```python
from build123d import *

# Parameters (mm, degrees)
BOSS_EXTRUDE1_DEPTH      = 150
BOSS_EXTRUDE1_DEPTH_BACK = 150
SKETCH2_W                = 600
SKETCH2_H                = 200
SKETCH3_W                = 200
SKETCH3_H                = 100
CUT_EXTRUDE1_DEPTH       = 100
SKETCH4_W                = 25
SKETCH4_H                = 25
BOSS_EXTRUDE2_DEPTH      = 5
MIRROR3_COPY_1_SKETCH_W  = 25
MIRROR3_COPY_1_SKETCH_H  = 25
MIRROR3_COPY_1_DEPTH     = 5
CUT_EXTRUDE3_DEPTH       = 200


with BuildPart() as part:
    # Sketch2 → Boss-Extrude1 (new, two sides: drawn at the far end of the back side and taken through both)
    with BuildSketch(Plane(origin=(0, 0, 0), x_dir=(0, 0, -1), z_dir=(1, 0, 0)).offset(-BOSS_EXTRUDE1_DEPTH_BACK)):
        Rectangle(SKETCH2_W, SKETCH2_H)
    extrude(amount=BOSS_EXTRUDE1_DEPTH + BOSS_EXTRUDE1_DEPTH_BACK)

    # Sketch3 → Cut-Extrude1 (cut)
    with BuildSketch(Plane(origin=(150, 0, 0), x_dir=(0, 0, -1), z_dir=(1, 0, 0))):
        with Locations((-200, -50)):
            Rectangle(SKETCH3_W, SKETCH3_H)
        with Locations((200, -50)):
            Rectangle(SKETCH3_W, SKETCH3_H)
    cut_extrude1 = extrude(amount=-CUT_EXTRUDE1_DEPTH, mode=Mode.SUBTRACT)

    # Mirror1: Cut-Extrude1 across plane
    add(cut_extrude1.mirror(Plane(origin=(0, 0, 0), x_dir=(0, 0, 1), z_dir=(1, 0, 0))), mode=Mode.SUBTRACT)

    # Sketch4 → Boss-Extrude2 (add)
    with BuildSketch(Plane.XZ):
        with Locations((112.5, 212.5)):
            Rectangle(SKETCH4_W, SKETCH4_H)
    boss_extrude2 = extrude(amount=BOSS_EXTRUDE2_DEPTH)

    # Mirror2: Boss-Extrude2 across plane
    add(boss_extrude2.mirror(Plane(origin=(0, 0, 0), x_dir=(0, 0, 1), z_dir=(1, 0, 0))))

    # Mirror3: Boss-Extrude2 across plane
    add(boss_extrude2.mirror(Plane.XY))

    # Mirror3 copy 1 sketch → Mirror3 copy 1 (add)
    with BuildSketch(Plane(origin=(0, 0, 0), x_dir=(-1, 0, 0), z_dir=(0, -1, 0))):
        with Locations((112.5, 212.5)):
            Rectangle(MIRROR3_COPY_1_SKETCH_W, MIRROR3_COPY_1_SKETCH_H)
    extrude(amount=MIRROR3_COPY_1_DEPTH)

    # Sketch5 → Cut-Extrude3 (cut)
    with BuildSketch(Plane(origin=(0, 0, -300), x_dir=(-1, 0, 0), z_dir=(0, 0, -1))):
        Polygon((-20, -100), (-50, 0), (-50, -100), align=None)
        Polygon((50, -100), (50, 0), (20, -100), align=None)
    cut_extrude3 = extrude(amount=-CUT_EXTRUDE3_DEPTH, mode=Mode.SUBTRACT)

    # Mirror4: Cut-Extrude3 across plane
    add(cut_extrude3.mirror(Plane.XY), mode=Mode.SUBTRACT)


solid = part.part
```
Model file for the job. Use its own axes, mm. A direction names the side the tool comes from. Coordinates: 2 decimals unless noted, no trailing zeros. Loops run counter-clockwise (first coordinate to the right, second up) from the corner with the lowest first, then second, coordinate; pieces in that order, holes last. Notation, with made-up numbers: (-33.5, 22.5) - (-1.5, 22.5) arc R11 ccw to (-1.5, 28.5) - close; hole circle Ø5 at (-17, 6). An arc over 180 degrees is marked (long way). Write item = value, one per line. Start each with the question number.
Item 1: 3-axis set-ups, long thin cutter, end or side, ignore diameter. For faces 5 (the face through (-112, -5, 213)), 6 (the face through (-2, -100, 4)), 7 (the face through (112, -5, -213)), 8 (the face through (-2, 100, 4)), 9 (the face through (112, -5, 213)): which of +Z, -Z, +X, -X, +Y, -Y reach the whole face in a straight line?
Item 2: Saw through at C-C, the plane x = 85. List the corners of the cut face in (y, z).
Item 3: Saw through at A-A, the plane z = -264. List the corners of the cut face in (x, y).
Item 4: Saw through at D-D, the plane y = -79. List the corners of the cut face in (x, z).
Item 5: Wall check: probe 1 along Y at (x, z) = (136, -265); probe 2 along Z at (x, y) = (-124, -39); probe 3 along X at (y, z) = (-35.5, 148). Give the ranges that are in metal, low to high. Write a range as [from, to].
Item 6: Drop flat-ended pins along their axis: pin 1 Ø1.5 at (x, y) = (108.5, -17.5) entering from +Z; pin 2 Ø4 at (x, y) = (-108.5, -3.5) entering from +Z; pin 3 Ø1.5 at (y, z) = (-3, 211) entering from -X. Give the stop position or say it passes through.
Item 7: Saw through at B-B, the plane y = -11. List the corners of the cut face in (x, z).
Item 8: Pull direction Z, two halves, no side cores. Call faces 1 (the face through (-101, 0, -199)), 2 (the face through (-2, 43, 300)), 3 (the face through (-150, 24, 4)), 4 (the face through (90, 0, 201)): +Z half, -Z half, draft (parallel to the pull), parting line (faces both ways), or undercut.
Answers:
q1.face_5 = +Z, -X, -Y
q1.face_6 = +Z, -Z, +X, -X, -Y
q1.face_7 = -Z, +X, -Y
q1.face_8 = +Z, -Z, +X, -X, +Y
q1.face_9 = +Z, +X, -Y
q2.outline = (-100, -100) - (0, -100) - (0, -300) - (100, -300) - (100, 300) - (0, 300) - (0, 100) - (-100, 100) - close
q3.outline = (-150, 0) - (-50, 0) - (-20, -100) - (20, -100) - (50, 0) - (150, 0) - (150, 100) - (-150, 100) - close
q4.outline = (-150, -100) - (-26.3, -100) - (-26.3, -300) - (26.3, -300) - (26.3, -100) - (150, -100) - (150, 100) - (26.3, 100) - (26.3, 300) - (-26.3, 300) - (-26.3, 100) - (-150, 100) - close
q5.probe_1 = [0, 100]
q5.probe_2 = [-100, 100]
q5.probe_3 = [-39.35, 39.35]
q6.pin_1 = 100
q6.pin_2 = 225
q6.pin_3 = -125
q7.outline = (-150, -100) - (-46.7, -100) - (-46.7, -300) - (46.7, -300) - (46.7, -100) - (150, -100) - (150, 100) - (46.7, 100) - (46.7, 300) - (-46.7, 300) - (-46.7, 100) - (-150, 100) - close
q8.face_1 = undercut
q8.face_2 = +Z half
q8.face_3 = draft
q8.face_4 = undercut
